Autodesk Fusion 360 part; units mm, degrees
sketch "Schizzo1" plane through (0, 0, 0) normal (0, 0, 1) x (1, 0, 0)
  circle A0 centre (0, 0) radius 1
  dimension "d1" = 2
extrude "Estrudi1" add sketch "Schizzo1" along normal blind 37.9
sketch "Schizzo2" plane through (0, 0, 0) normal (0, 1, 0) x (1, 0, 0)
sketch "Schizzo3" plane through (0, 0, 0) normal (0, 0, 1) x (1, 0, 0)
  line L0 (-2.9326, -3.8) -> (2.9326, -3.8)
  arc A0 (2.9326, -3.8) -> (-2.9326, -3.8) centre (0, 0) ccw
  point P0 (0, 4.8)
  dimension "d4" = 9.6
  dimension "d6" = 3.8
  dimension "d7" = 8.6
extrude "Estrudi2" add sketch "Schizzo3" along normal blind 2.4 from surface at 1
sketch "Schizzo4" plane through (0, 0, 3.4) normal (0, 0, 1) x (-1, 0, 0)
  arc A0 (-2.9326, 3.8) -> (2.9326, 3.8) centre (0, 0) ccw
  line L0 (2.9326, 3.8) -> (-2.9326, 3.8)
  circle A1 centre (0, 0) radius 1
  line L1 (6.4622, -7.5) -> (-6.4622, -7.5)
  line L2 (-6.4622, 7.5) -> (6.4622, 7.5)
  arc A2 (-6.4622, 7.5) -> (-6.4622, -7.5) centre (0, 0) ccw
  arc A3 (6.4622, -7.5) -> (6.4622, 7.5) centre (0, 0) ccw
  dimension "d11" = 19.8
  dimension "d12" = 7.5
  dimension "d21" = 15
extrude "Estrudi3" add sketch "Schizzo4" along normal blind 25 contours A0 L0 | L1 L2 A2 A3
sketch "Schizzo5" plane through (0, 0, 28.4) normal (0, 0, 1) x (-1, 0, 0)
  circle A0 centre (0, 0) radius 1
  arc A1 (-6.4622, 7.5) -> (-6.4622, -7.5) centre (0, 0) ccw
  line L0 (-6.4622, -7.5) -> (6.4622, -7.5)
  arc A2 (6.4622, -7.5) -> (6.4622, 7.5) centre (0, 0) ccw
  line L1 (6.4622, 7.5) -> (-6.4622, 7.5)
  circle A3 centre (0, 0) radius 2.8
  dimension "d16" = 5.6
extrude "Estrudi4" add sketch "Schizzo5" along normal blind 1.6 contours A3
fillet "Raccordo1" radius 1 4 faces at (-2.1541, 7.5, 11.7333) (2.1541, -7.5, 11.7333) (7.7686, 6.1367, 20.0667) (-7.7686, -6.1367, 20.0667)
equation "d9 = 3.4 mm - 1 mm"
equation "d12 = ( 15 / 2 ) * 1 mm"
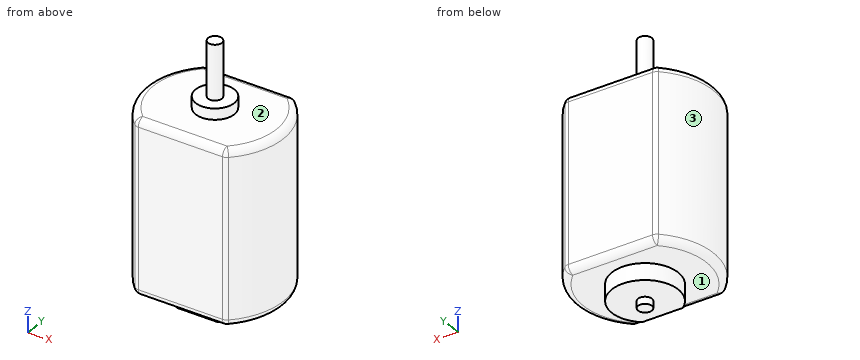
Verification items for the finished model (mm, model axes). Face numbers are marked on the shaded views. A direction names the side the tool comes from. Give positions to 0.01 mm unless a question says otherwise; leave off trailing zeros. Order: outer loops, then holes, each group sorted by start corner. A loop starts at its lowest first (then second) coordinate and runs counter-clockwise, first axis right, second up. Notation, with made-up numbers: (39, 83.25) -> (94, 83.25) arc R25 ccw to (94, 108.25) -> close; hole circle Ø10 at (29.25, 89.5). An arc over 180 degrees is marked (long way). Use a Markdown table: item, result.
1) Section check C-C, the plane z = 34. Record the boundary of the cut face in (x, y), then the cut area to 3 significant figures.
Results:
| item | result |
|---|---|
| outline | circle Ø2 at (0, 0) |
| area | 3.14 mm² |
2) Section check A-A, the plane x = 0. Record the boundary of the cut face in (y, z).
Results:
| item | result |
|---|---|
| outline | (-7.5, 4.4) arc R1 ccw to (-6.5, 3.4) -> (-3.8, 3.4) -> (-3.8, 1) -> (-1, 1) -> (-1, 0) -> (1, 0) -> (1, 1) -> (4.8, 1) -> (4.8, 3.4) -> (6.5, 3.4) arc R1 ccw to (7.5, 4.4) -> (7.5, 27.4) arc R1 ccw to (6.5, 28.4) -> (2.8, 28.4) -> (2.8, 30) -> (1, 30) -> (1, 37.9) -> (-1, 37.9) -> (-1, 30) -> (-2.8, 30) -> (-2.8, 28.4) -> (-6.5, 28.4) arc R1 ccw to (-7.5, 27.4) -> close |
3) Section check D-D, the plane x = -2.25. Record the boundary of the cut face in (y, z), then the cut area to 3 significant figures.
Results:
| item | result |
|---|---|
| outline | (-7.5, 4.4) arc R1 ccw to (-6.5, 3.4) -> (-3.8, 3.4) -> (-3.8, 1) -> (4.24, 1) -> (4.24, 3.4) -> (6.5, 3.4) arc R1 ccw to (7.5, 4.4) -> (7.5, 27.4) arc R1 ccw to (6.5, 28.4) -> (1.67, 28.4) -> (1.67, 30) -> (-1.67, 30) -> (-1.67, 28.4) -> (-6.5, 28.4) arc R1 ccw to (-7.5, 27.4) -> close |
| area | 399 mm² |
4) Section check B-B, the plane y = 0. Record the boundary of the cut face in (x, z), then the cut area to 3 significant figures.
Results:
| item | result |
|---|---|
| outline | (-9.9, 4.4) arc R1 ccw to (-8.9, 3.4) -> (-4.8, 3.4) -> (-4.8, 1) -> (-1, 1) -> (-1, 0) -> (1, 0) -> (1, 1) -> (4.8, 1) -> (4.8, 3.4) -> (8.9, 3.4) arc R1 ccw to (9.9, 4.4) -> (9.9, 27.4) arc R1 ccw to (8.9, 28.4) -> (2.8, 28.4) -> (2.8, 30) -> (1, 30) -> (1, 37.9) -> (-1, 37.9) -> (-1, 30) -> (-2.8, 30) -> (-2.8, 28.4) -> (-8.9, 28.4) arc R1 ccw to (-9.9, 27.4) -> close |
| area | 544 mm² |
5) Depth check by flat-ended pin: pin 1 Ø1.5 at (y, z) = (-3, 7.5) entering from -X; pin 2 Ø1.5 at (y, z) = (-1.5, 17) entering from -X; pin 3 Ø1.5 at (x, y) = (3, -1) entering from -Z. Enter the tip coordinate at first touch or a pass-through.
Results:
| item | result |
|---|---|
| pin 1 | x = -9.64 |
| pin 2 | x = -9.87 |
| pin 3 | z = 1 |
6) Tool access check on the marked faces 1, 2 and 3. Record the directions out of +Z, -Z, +X, -X, +Y, -Y that give a thin tool (end or side, any length) a straight path to the whole face; none if there is none.
Results:
| item | result |
|---|---|
| face 1 | -Z |
| face 2 | +Z |
| face 3 | +Z, -Z, -X |
7) Material ranges on probe 1 along Z at (x, y) = (3, -5.5); probe 2 along Z at (x, y) = (-2.5, 3); probe 3 along Y at (x, z) = (-8.75, 22), recorded low to high.
Results:
| item | result |
|---|---|
| probe 1 | 3.4 to 28.4 |
| probe 2 | 1 to 28.4 |
| probe 3 | -4.63 to 4.63 |
